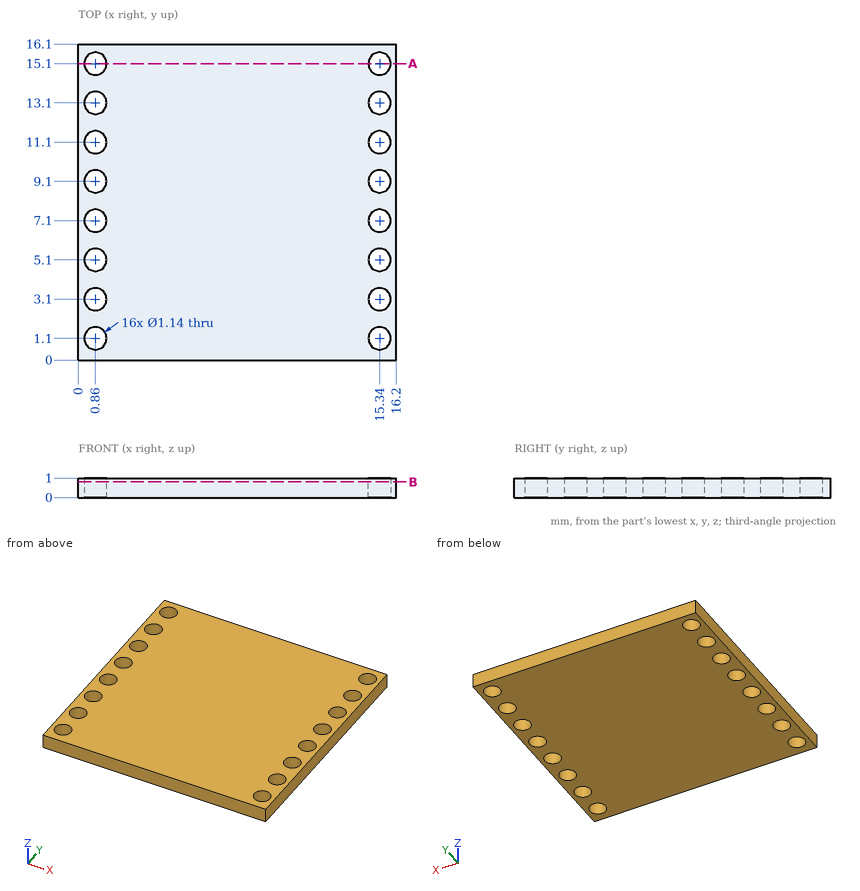
Print and shaded views of the part. All mm, measured from the part's lowest x, y and z. Round coordinates to 2 decimals unless told otherwise and drop trailing zeros. Order: outer loops, then holes, each group sorted by start corner. A loop starts at its lowest first (then second) coordinate and runs counter-clockwise, first axis right, second up.
Q1. Slice it at B-B (z = 0.8). State how many separate pieces and enclosed holes the cut face has, and give its area (3 significant figures).
Q2. Slice it at A-A (y = 15.1). Write the cut outline in (x, z).
Q3. Wall check: L1, parallel to X at y = 5.5, z = 0.35; L2, parallel to X at y = 1.25, z = 0.15. Give the ranges that are in metal, low to high.
Results below:
1. separate pieces: 1
1. enclosed holes: 16
1. area: 244 mm2
2. outline: (0, 0) - (0.29, 0) - (0.29, 1) - (0, 1) - close; (1.43, 0) - (14.77, 0) - (14.77, 1) - (1.43, 1) - close; (15.91, 0) - (16.2, 0) - (16.2, 1) - (15.91, 1) - close
3. L1: x = 0 to 0.45, 1.27 to 14.93, 15.75 to 16.2
3. L2: x = 0 to 0.31, 1.41 to 14.79, 15.89 to 16.2
